from build123d import *

# Parameters (mm, degrees)
F0_R      = 7.85
F0_R_2    = 4.39
F1_DEPTH  = 6
F2_R      = 5.5
F2_R_2    = 4.39
F3_DEPTH  = 1.95
F4_R      = 7.85
F4_R_2    = 5.5
F5_DEPTH  = 9.5
F6_DEPTH  = 9.5
F8_R      = 5.5
F8_R_2    = 4.39
F9_DEPTH  = 1.95
F10_R     = 7.85
F10_R_2   = 5.5
F10_R_3   = 4.39
F11_DEPTH = 6
F12_SIZE  = 1
F13_SIZE  = 1


with BuildPart() as f1:
    # F0 (on Top) → F1 (new body)
    with BuildSketch(Plane.XY):
        Circle(F0_R)
        Circle(F0_R_2, mode=Mode.SUBTRACT)
    extrude(amount=F1_DEPTH)

    # F2 (on face) → F3 (join)
    with BuildSketch(Plane.XY.offset(6)):
        Circle(F2_R)
        Circle(F2_R_2, mode=Mode.SUBTRACT)
    extrude(amount=F3_DEPTH)


with BuildPart() as f5:
    # F4 (on face) → F5 (new body)
    with BuildSketch(Plane.XY.offset(7.95)):
        Circle(F4_R)
        Circle(F4_R_2, mode=Mode.SUBTRACT)
    extrude(amount=F5_DEPTH)


with BuildPart() as f6:
    # F6 (new): a face of the model
    f6_faces = [f1.part.faces().sort_by_distance(p)[0] for p in [
        (-5.3444365081, 0, 7.95),
    ]]
    extrude(f6_faces, amount=F6_DEPTH)


with BuildPart() as f1_1:
    add(f1.part)

    # F7: union F5, F6
    add(f5.part)
    add(f6.part)

    # F8 (on face) → F9 (join)
    with BuildSketch(Plane.XY.offset(17.45)):
        Circle(F8_R)
        Circle(F8_R_2, mode=Mode.SUBTRACT)
    extrude(amount=F9_DEPTH)

    # F10 (on face) → F11 (join)
    with BuildSketch(Plane.XY.offset(19.4)):
        Circle(F10_R)
        Circle(F10_R_2, mode=Mode.SUBTRACT)
        Circle(F10_R_2)
        Circle(F10_R_3, mode=Mode.SUBTRACT)
    extrude(amount=F11_DEPTH)

    # F12
    f12_edges = [f1_1.edges().sort_by_distance(p)[0] for p in [
        (-7.85, 0, 25.4),
    ]]
    chamfer(f12_edges, length=F12_SIZE)

    # F13
    f13_edges = [f1_1.edges().sort_by_distance(p)[0] for p in [
        (-7.85, 0, 0),
    ]]
    chamfer(f13_edges, length=F13_SIZE)


solid = f1_1.part
Design review of the part built by this model. Coordinates are the model's own, in mm. A direction names the side the tool comes from. Coordinates: 2 decimals unless noted, no trailing zeros. Write each loop counter-clockwise with the first axis right and the second up, starting at its lowest first coordinate (ties: lowest second). Pieces come first, ordered by that corner, then holes. Notation, with made-up numbers: (86, 63) - (136, 63) arc R27 cw to (136, 84) - close; hole circle Ø5 at (59, -3.5). An arc over 180 degrees is marked (long way). One line per item, written item: value.
1) To check wall thickness, follow probe 1 along Z at (x, y) = (2.5, -5.5); probe 2 along Z at (x, y) = (6, 4.75); probe 3 along Y at (x, z) = (-0.25, 17.5). State the ranges of each line that lie inside material, in increasing order.
Answer sheet:
probe 1: z = 0 to 6, 7.95 to 17.45, 19.4 to 25.4
probe 2: z = 0.8 to 6, 7.95 to 17.45, 19.4 to 24.6
probe 3: y = -5.49 to -4.38, 4.38 to 5.49
2) Add section D-D (y = -6.5). Give the number of separate pieces and of enclosed holes in the cut face, plus the area to 3 significant figures.
Answer sheet:
separate pieces: 3
enclosed holes: 0
area: 185 mm2
3) Add section A-A (y = 0). State the section outline as (x, z) points.
Answer sheet:
outline: (-7.85, 1) - (-6.85, 0) - (-4.39, 0) - (-4.39, 25.4) - (-6.85, 25.4) - (-7.85, 24.4) - (-7.85, 19.4) - (-5.5, 19.4) - (-5.5, 17.45) - (-7.85, 17.45) - (-7.85, 7.95) - (-5.5, 7.95) - (-5.5, 6) - (-7.85, 6) - close; (4.39, 0) - (6.85, 0) - (7.85, 1) - (7.85, 6) - (5.5, 6) - (5.5, 7.95) - (7.85, 7.95) - (7.85, 17.45) - (5.5, 17.45) - (5.5, 19.4) - (7.85, 19.4) - (7.85, 24.4) - (6.85, 25.4) - (4.39, 25.4) - close
4) For faces 1 (the face through (-1.85, 5.34, 6)), 2 (the face through (-5.786, 5.305, 3.465)), list the 3-axis set-ups (+Z, -Z, +X, -X, +Y, -Y) from which the entire face can be reached by the end or side of a thin tool; tool diameter is ignored.
Answer sheet:
face 1: none
face 2: +Z, -Z
5) Add section C-C (z = 14.75). State the section outline as (x, y) points, plus the area to 3 significant figures.
Answer sheet:
outline: circle Ø15.7 at (0, 0); hole circle Ø8.78 at (0, 0)
area: 133 mm2
6) Insertion check: pin 1 (8 mm diameter, centred on x = -0.5, z = 9, fed in from -Y); pin 2 (2 mm diameter, centred on x = -4.5, z = 22, fed in from +Y); pin 3 (6 mm diameter, centred on x = -5, z = 7, fed in from -Y); pin 4 (1.5 mm diameter, centred on x = -5.5, y = 6, fed in from -Z). Each pin has a flat end and moves straight along its axis. Give the tip position at first contact, or say it passes through.
Answer sheet:
pin 1: stops at y = -7.85
pin 2: stops at y = 7.03
pin 3: stops at y = -7.55
pin 4: stops at z = 0.54
7) Mouldability with a two-part tool opening along Z and no side actions: class faces 3 (the face through (-1.19, -5.37, 18.41)), 4 (the face through (4.5, -1.4, 25.4)), 5 (the face through (-0.571, 4.353, 12.522)) as +Z half, -Z half, draft (parallel to the pull), parting line (faces both ways), or undercut.
Answer sheet:
face 3: undercut
face 4: +Z half
face 5: draft
